Verification items for the finished model (mm, model axes). A direction names the side the tool comes from. Round coordinates to 2 decimals unless told otherwise and drop trailing zeros. Order: outer loops, then holes, each group sorted by start corner. A loop starts at its lowest first (then second) coordinate and runs counter-clockwise, first axis right, second up. Notation, with made-up numbers: (72.25, 62.25) -> (79.25, 62.25) arc R22 cw to (79.25, 93.25) -> close; hole circle Ø2 at (50.5, 19.25). An arc over 180 degrees is marked (long way). Answer in a Markdown table with one row per item. Add a question column.
```python
from build123d import *

# Parameters (mm, degrees)
SKETCH1_R           = 1.397
BOSS_EXTRUDE1_DEPTH = 3.175
SKETCH2_W           = 31.75
SKETCH2_H           = 12.7
SKETCH2_R           = 2.0193
BOSS_EXTRUDE2_DEPTH = 3.175
FILLET1_R           = 1.27
FILLET2_R           = 2.54


with BuildPart() as part:
    # Sketch1 → Boss-Extrude1 (new body)
    with BuildSketch(Plane.XY):
        with BuildLine():
            Line((-4.0005, 13.208), (-4.0005, 15.875))
            Line((-4.0005, 15.875), (-15.875, 15.875))
            Line((-15.875, 15.875), (-15.875, 0))
            Line((-15.875, 0), (15.875, 0))
            Line((15.875, 0), (15.875, 15.875))
            Line((15.875, 15.875), (4.0005, 15.875))
            Line((4.0005, 15.875), (4.0005, 13.208))
            ThreePointArc((4.0005, 13.208), (0, 9.2075), (-4.0005, 13.208))
        make_face()
        with Locations((12.446, 13.208)):
            Circle(SKETCH1_R, mode=Mode.SUBTRACT)
        with Locations((-12.446, 13.208)):
            Circle(SKETCH1_R, mode=Mode.SUBTRACT)
    extrude(amount=-BOSS_EXTRUDE1_DEPTH)

    # Sketch2 → Boss-Extrude2 (add)
    with BuildSketch(Plane(origin=(0, 0, 0), x_dir=(1, 0, 0), z_dir=(0, 1, 0))):
        with Locations((0, -6.35)):
            Rectangle(SKETCH2_W, SKETCH2_H)
        with Locations(Location((-9.525, -6.35, 0), (0, 0, 270))):
            Circle(SKETCH2_R, mode=Mode.SUBTRACT)
        with Locations(Location((9.525, -6.35, 0), (0, 0, 270))):
            Circle(SKETCH2_R, mode=Mode.SUBTRACT)
    extrude(amount=BOSS_EXTRUDE2_DEPTH)

    # Fillet1
    fillet1_edges = [part.edges().sort_by_distance(p)[0] for p in [
        (0, 3.175, 0),
    ]]
    fillet(fillet1_edges, radius=FILLET1_R)

    # Fillet2
    fillet2_edges = [part.edges().sort_by_distance(p)[0] for p in [
        (0, 0, -3.175),
    ]]
    fillet(fillet2_edges, radius=FILLET2_R)


solid = part.part
```
1) Cross-section at B-B, the plane y = 15.25. Record the boundary of the cut face in (x, z) (1 decimal), and give its area (3 significant figures).
2) Thickness scan on L1, parallel to X at y = 2.35, z = 6.35 (3 decimals); L2, parallel to Z at x = 10, y = 13.25 (3 decimals); L3, parallel to Y at x = 14.5, z = 5.75 (3 decimals). Record the ranges inside material, lowest first. Write a range as [from, to].
3) Cross-section at C-C, the plane x = 6. Record the boundary of the cut face in (y, z) (3 decimals), and give its area (3 significant figures).
4) Cross-section at D-D, the plane x = 12.5. Record the boundary of the cut face in (y, z) (3 decimals), and give its area (3 significant figures).
5) Draft check along X on faces 4 (the face through (0, 9, 0)), 5 (the face through (-15.875, 3, 1)), 6 (the face through (15.875, 3, 1)), 7 (the face through (4, 15, -2)). Enter one of: +X half, -X half, draft (parallel to the pull), parting line (faces both ways), or undercut.
6) Tool access check on faces 1 (the face through (0, 0, 6)), 2 (the face through (0, 3.175, 7)), 3 (the face through (-4, 15, -2)). Record the directions out of +Z, -Z, +X, -X, +Y, -Y that give a thin tool (end or side, any length) a straight path to the whole face; none if there is none.
7) Depth check by flat-ended pin: P1, Ø5.5, axis at x = -3.5, y = 10, coming from the +Z side. Enter the tip coordinate at first touch or a pass-through.
8) Cross-section at A-A, the plane z = 6.35. Record the boundary of the cut face in (x, y) (3 decimals), and give its area (3 significant figures).
Results below:
| question | item | result |
|---|---|---|
| 1 | outline | (-15.9, -3.2) -> (-4, -3.2) -> (-4, 0) -> (-15.9, 0) -> close; (4, -3.2) -> (15.9, -3.2) -> (15.9, 0) -> (4, 0) -> close |
| 1 | area | 75.4 mm² |
| 2 | L1 | [-15.875, -11.544], [-7.506, 7.506], [11.544, 15.875] |
| 2 | L2 | [-3.175, 0] |
| 2 | L3 | [0, 3.175] |
| 3 | outline | (0, -0.635) arc R2.54 ccw to (2.54, -3.175) -> (15.875, -3.175) -> (15.875, 0) -> (4.445, 0) arc R1.27 cw to (3.175, 1.27) -> (3.175, 12.7) -> (0, 12.7) -> close |
| 3 | area | 89.7 mm² |
| 4 | outline | (0, -0.635) arc R2.54 ccw to (2.54, -3.175) -> (11.812, -3.175) -> (11.812, 0) -> (4.445, 0) arc R1.27 cw to (3.175, 1.27) -> (3.175, 12.7) -> (0, 12.7) -> close; (14.604, -3.175) -> (15.875, -3.175) -> (15.875, 0) -> (14.604, 0) -> close |
| 4 | area | 80.8 mm² |
| 5 | face 4 | draft |
| 5 | face 5 | -X half |
| 5 | face 6 | +X half |
| 5 | face 7 | undercut |
| 6 | face 1 | +Z, -Z, +X, -X, -Y |
| 6 | face 2 | +Z, +X, -X, +Y |
| 6 | face 3 | +Z, -Z, +Y |
| 7 | P1 | z = 0 |
| 8 | outline | (-15.875, 0) -> (-11.544, 0) -> (-11.544, 3.175) -> (-15.875, 3.175) -> close; (-7.506, 0) -> (7.506, 0) -> (7.506, 3.175) -> (-7.506, 3.175) -> close; (11.544, 0) -> (15.875, 0) -> (15.875, 3.175) -> (11.544, 3.175) -> close |
| 8 | area | 75.2 mm² |
